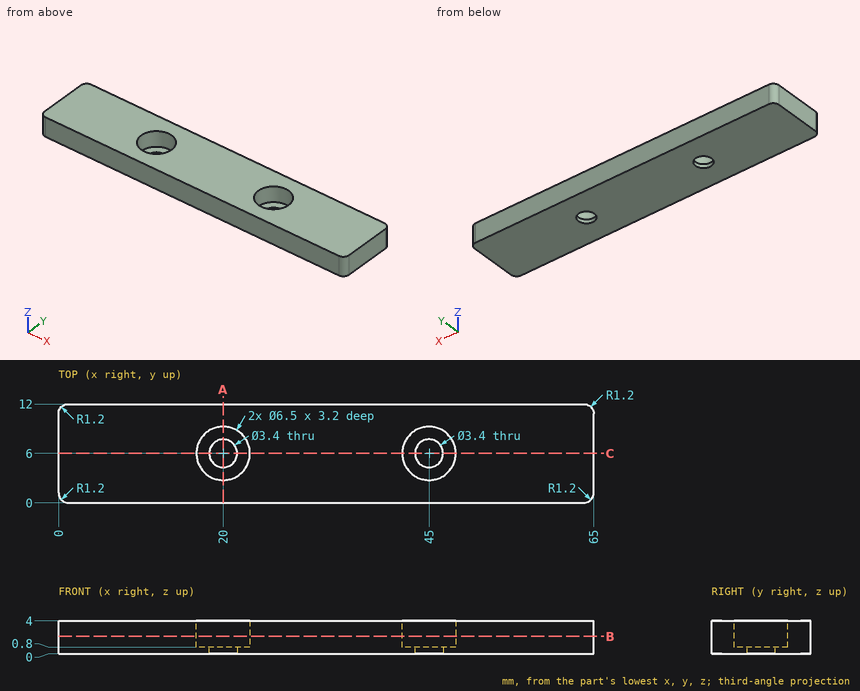
Source: three-view drawing plus pictorial views. Frame: mm from the lowest corner of the part. Give positions to 0.01 mm unless a question says otherwise; leave off trailing zeros. Write each loop counter-clockwise with the first axis right and the second up, starting at its lowest first coordinate (ties: lowest second). Pieces come first, ordered by that corner, then holes.
(1) Cut plane B-B, the plane z = 2.1. Return loops of the section in (x, y), then the cut area to 3 significant figures.
(2) Ray query, line 1 (X direction, y = 6.25, z = 1.2); line 2 (Y direction, x = 20, z = 2.5); line 3 (X direction, y = 4.5, z = 3.25). Return the intervals inside material, ascending.
(3) Cut plane A-A, the plane x = 20. Return loops of the section in (y, z).
(4) Cut plane C-C, the plane y = 6. Return loops of the section in (x, z), then the cut area to 3 significant figures.
(5) First-contact query: P1, Ø4, axis at x = 20, y = 6, coming from the +Z side. Flat tip, straight axial feed; report the tip coordinate or a pass-through.
Values follow:
1. outline: (0, 1.2) arc R1.2 ccw to (1.2, 0) - (63.8, 0) arc R1.2 ccw to (65, 1.2) - (65, 10.8) arc R1.2 ccw to (63.8, 12) - (1.2, 12) arc R1.2 ccw to (0, 10.8) - close; hole circle Ø6.5 at (20, 6); hole circle Ø6.5 at (45, 6)
1. area: 712 mm2
2. line 1: x = 0 to 16.76, 23.24 to 41.76, 48.24 to 65
2. line 2: y = 0 to 2.75, 9.25 to 12
2. line 3: x = 0 to 17.12, 22.88 to 42.12, 47.88 to 65
3. outline: (0, 0) - (4.3, 0) - (4.3, 0.8) - (2.75, 0.8) - (2.75, 4) - (0, 4) - close; (7.7, 0) - (12, 0) - (12, 4) - (9.25, 4) - (9.25, 0.8) - (7.7, 0.8) - close
4. outline: (0, 0) - (18.3, 0) - (18.3, 0.8) - (16.75, 0.8) - (16.75, 4) - (0, 4) - close; (21.7, 0) - (43.3, 0) - (43.3, 0.8) - (41.75, 0.8) - (41.75, 4) - (23.25, 4) - (23.25, 0.8) - (21.7, 0.8) - close; (46.7, 0) - (65, 0) - (65, 4) - (48.25, 4) - (48.25, 0.8) - (46.7, 0.8) - close
4. area: 213 mm2
5. P1: stops at z = 0.8
